Build history of the part. All positions in model axes, mm. A direction names the side the tool comes from. Round coordinates to 2 decimals unless told otherwise and drop trailing zeros. Write each loop counter-clockwise with the first axis right and the second up, starting at its lowest first coordinate (ties: lowest second). Pieces come first, ordered by that corner, then holes. Notation, with made-up numbers: (81.5, -30.75) -> (107.5, -30.75) arc R25 cw to (107.5, 8.25) -> close; hole circle Ø6 at (63.25, 43.5). An arc over 180 degrees is marked (long way). Return JSON: item names as keys, results as strings.
Autodesk Inventor part; units mm, degrees
ref_plane "YZ Plane" through (0, 0, 0) normal (1, 0, 0) x (0, 1, 0)
ref_plane "XZ Plane" through (0, 0, 0) normal (0, 1, 0) x (-1, 0, 0)
ref_plane "XY Plane" through (0, 0, 0) normal (0, 0, 1) x (1, 0, 0)
sketch "эскиз_корпус" plane through (0, 0, 0) normal (0, 0, 1) x (1, 0, 0)
  line L0 (0.9426, 4.9612) -> (-0.95, -5)
  line L1 (-5.05, 0) -> (5.05, 0)
  arc A0 (5.05, 0) -> (-5.05, 0) centre (0, 0) ccw
  line L2 (-5.05, 0) -> (-5.05, -5)
  line L3 (5.05, 0) -> (5.05, -5)
  arc A1 (5, 0) -> (-5, 0) centre (0, 0) ccw
  line L4 (-5.05, -5) -> (-5, -5)
  line L5 (5, -5) -> (5.05, -5)
  line L6 (5.05, -5) -> (25.05, -5)
  line L7 (-25.05, -5) -> (-5.05, -5)
  line L8 (-0.95, -5) -> (5, -5)
  line L9 (-0.95, -5) -> (-5, -5)
  line L10 (5, -5) -> (5, 0)
  line L11 (-5, 0) -> (-5, -5)
  line L12 (25.05, -5) -> (25.05, -15)
  line L13 (25.05, -15) -> (-25.05, -15)
  line L14 (-25.05, -15) -> (-25.05, -5)
  dimension "d33" = 5
  dimension "d34" = 5
  dimension "d52" = 0.05
  dimension "d85" = 10
  dimension "d89" = 20
  dimension "d91" = 20
extrude "корпус_общий" add sketch "эскиз_корпус" along normal blind 80
sketch "эскиз_отверстие_ручка" plane through (-5.05, -5, 0) normal (-1, 0, 0) x (0, 0, 1)
  line L0 (0, 0) -> (80, 0)
  line L1 (0, 5) -> (80, 5)
  line L2 (13.9957, 20) -> (13.9957, 0)
  line L3 (0, 0) -> (80, 0)
  line L4 (13.9957, 20) -> (33.9957, 20)
  line L5 (33.9957, 20) -> (33.9957, 0)
  line L6 (28.9957, 0) -> (28.9957, 7.5)
  line L7 (28.9957, 7.5) -> (18.9957, 7.5)
  line L8 (18.9957, 7.5) -> (18.9957, 0)
  line L9 (0, 5) -> (0, 5)
  line L10 (0, 5) -> (80, 5)
  line L11 (80, 5) -> (80, 5)
  line L12 (0, 5) -> (80, 5)
  line L13 (0, 10.05) -> (80, 10.05)
  line L14 (0, 5) -> (0, 10.05)
  line L15 (80, 5) -> (80, 10.05)
  dimension "d77" = 5
  dimension "d78" = 5
  dimension "d79" = 10
  dimension "d87" = 12.5
  dimension "d92" = 20
extrude "отверстие_ручка" cut sketch "эскиз_отверстие_ручка" against normal blind 7.5 contours L2 L1 L8 L0 | L2 L13 L5 L1 L6 L7 L8 | L6 L1 L5 L0 | L2 L4 L5 L13
extrude "отверстие_цилиндр" cut sketch "эскиз_корпус" along normal blind 80 contours A1 L1 L0 | L0 L1 A1 | L1 L10 L8 L0 | L0 L9 L11 L1
equation "\"d33\" = diametr_ruchka_"
equation "\"d34\" = diametr_ruchka_"
equation "\"d85\" = diametr_"
equation "\"d89\" = 2 * diametr_"
equation "\"d91\" = 2 * diametr_"
equation "\"d74\" = length"
equation "\"d77\" = diametr_ruchka_"
equation "\"d78\" = diametr_ruchka_"
equation "\"d79\" = diametr_"
equation "\"d87\" = 2.5 * diametr_ruchka_"
equation "\"d92\" = 2 * diametr_"
equation "\"d81\" = 1.5 * diametr_ruchka_"
equation "\"d83\" = length"
properties part number "lw_5_корпус_new"
Q1. Saw through at C-C on z = 73.5. List the corners of the cut face in (x, y).
Verdict:
{"outline": "(-25.05, -15) -> (25.05, -15) -> (25.05, -5) -> (5.05, -5) -> (5.05, 0) arc R5.05 ccw to (-5.05, 0) -> (-5.05, -5) -> (-25.05, -5) -> close; hole (-5, -5) -> (5, -5) -> (5, 0) arc R5 ccw to (-5, 0) -> close"}
Q2. Saw through at D-D on z = 20. List the corners of the cut face in (x, y).
Verdict:
{"outline": "(-25.05, -15) -> (25.05, -15) -> (25.05, -5) -> (5.05, -5) -> (5.05, 0) arc R5.05 ccw to (2.45, 4.42) -> (2.45, 4.36) arc R5 cw to (5, 0) -> (5, -5) -> (-5, -5) -> (-5, 0) arc R5 cw to (-4.33, 2.5) -> (-4.39, 2.5) arc R5.05 ccw to (-5.05, 0) -> (-5.05, -5) -> (-25.05, -5) -> close"}
Q3. Saw through at B-B on x = 0. List the corners of the cut face in (y, z), then the cut area to 3 significant figures.
Verdict:
{"outline": "(-15, 0) -> (-5, 0) -> (-5, 80) -> (-15, 80) -> close; (5, 0) -> (5.05, 0) -> (5.05, 14) -> (5, 14) -> close; (5, 34) -> (5.05, 34) -> (5.05, 80) -> (5, 80) -> close", "area": "803 mm²"}
Q4. Pin check, flat tips, straight feed: pin 1 Ø2.5 at (y, z) = (-1.5, 21.5) entering from -X; pin 2 Ø2.5 at (y, z) = (-3, 46.5) entering from +X; pin 3 Ø9 at (x, z) = (-8, 50) entering from +Y. Stop position of each tip, or through.
Verdict:
{"pin 1": "stops at x = -5.05", "pin 2": "stops at x = 5.05", "pin 3": "stops at y = 3.64"}
Q5. Saw through at A-A on y = -1.5. List the corners of the cut face in (x, z), then the cut area to 3 significant figures.
Verdict:
{"outline": "(-5.05, 0) -> (-5, 0) -> (-5, 14) -> (-5.05, 14) -> close; (-5.05, 19) -> (-5, 19) -> (-5, 29) -> (-5.05, 29) -> close; (-5.05, 34) -> (-5, 34) -> (-5, 80) -> (-5.05, 80) -> close; (5, 0) -> (5.05, 0) -> (5.05, 80) -> (5, 80) -> close", "area": "7.50 mm²"}
Q6. Two-plate mould, pull along X, no slides. Class faces 3 (the flat face through (-25.05, -10, 39)), 4 (the flat face through (-10, -5, 39)), 5 (the flat face through (0, -9, 0)): +X half, -X half, draft (parallel to the pull), parting line (faces both ways), or undercut.
Verdict:
{"face 3": "-X half", "face 4": "undercut", "face 5": "draft"}
Q7. 3-axis set-ups, long thin cutter, end or side, ignore diameter. For faces 1 (the flat face through (0, -9, 80)), 2 (the flat face through (15, -5, 39)): which of +Z, -Z, +X, -X, +Y, -Y reach the whole face in a straight line?
Verdict:
{"face 1": "+Z, +X, -X, +Y, -Y", "face 2": "+Z, -Z, +X, +Y"}
Q8. Wall check: L1, parallel to Y at x = -13, z = 71.5. Give the ranges that are in metal, low to high.
Verdict:
{"L1": "y = -15 to -5"}
